```python
from build123d import *

# Parameters (mm, degrees)
BOSS_EXTRUDE1_DEPTH = 6
BOSS_EXTRUDE4_DEPTH = 20
CUT_EXTRUDE2_DEPTH  = 15
CUT_EXTRUDE3_DEPTH  = 6
CHAMFER2_SIZE       = 2
CHAMFER2_SIZE2      = 3.464101615


with BuildPart() as part:
    # Sketch1 → Boss-Extrude1 (new body)
    with BuildSketch(Plane(origin=(0, 0, 0), x_dir=(1, 0, 0), z_dir=(0, 1, 0))):
        Polygon((16.25, 9.381941874), (0, 18.763883749), (-16.25, 9.381941874), (-16.25, -9.381941874), (0, -18.763883749), (16.25, -9.381941874), align=None)
        Polygon((11.25, 6.495190528), (0, 12.990381057), (-11.25, 6.495190528), (-11.25, -6.495190528), (0, -12.990381057), (11.25, -6.495190528), align=None, mode=Mode.SUBTRACT)
    extrude(amount=BOSS_EXTRUDE1_DEPTH)

    # Sketch5 → Boss-Extrude4 (add)
    with BuildSketch(Plane.XZ):
        Polygon((16.25, 9.381941874), (0, 18.763883749), (-16.25, 9.381941874), (-16.25, -9.381941874), (0, -18.763883749), (16.25, -9.381941874), align=None)
    extrude(amount=BOSS_EXTRUDE4_DEPTH)

    # Sketch6 → Cut-Extrude2 (cut)
    with BuildSketch(Plane.XZ.offset(20)):
        with BuildLine():
            Line((-2.618090908, 1.66), (-2.618090908, -1.66))
            ThreePointArc((-2.618090908, -1.66), (3.1, 0), (-2.618090908, 1.66))
        make_face()
    extrude(amount=-CUT_EXTRUDE2_DEPTH, mode=Mode.SUBTRACT)

    # Sketch7 → Cut-Extrude3 (cut)
    with BuildSketch(Plane(origin=(0, 6, 0), x_dir=(1, 0, 0), z_dir=(0, 1, 0))):
        Polygon((-6.495190528, 11.25), (-12.990381057, 0), (-6.495190528, -11.25), (6.495190528, -11.25), (12.990381057, 0), (6.495190528, 11.25), align=None)
    extrude(amount=-CUT_EXTRUDE3_DEPTH, mode=Mode.SUBTRACT)

    # Chamfer2
    chamfer2_edges = [part.edges().sort_by_distance(p)[0] for p in [
        (4.754809472, 6, 11.25),
        (7.365381057, 6, 9.742785793),
        (11.25, 6, 4.754809472),
        (9.742785793, 6, -7.365381057),
        (-1.507214207, 6, -12.120190528),
        (-11.25, 6, -4.754809472),
        (-9.742785793, 6, 7.365381057),
        (1.507214207, 6, 12.120190528),
        (9.742785793, 6, 7.365381057),
        (-1.507214207, 6, 12.120190528),
        (-11.25, 6, 4.754809472),
        (-9.742785793, 6, -7.365381057),
        (1.507214207, 6, -12.120190528),
        (11.25, 6, -4.754809472),
        (12.120190528, 6, 1.507214207),
        (12.120190528, 6, -1.507214207),
        (7.365381057, 6, -9.742785793),
        (4.754809472, 6, -11.25),
        (-4.754809472, 6, -11.25),
        (-7.365381057, 6, -9.742785793),
        (-12.120190528, 6, -1.507214207),
        (-12.120190528, 6, 1.507214207),
        (-7.365381057, 6, 9.742785793),
        (-4.754809472, 6, 11.25),
    ]]
    chamfer2_side = [part.faces().sort_by_distance(p)[0] for p in [
        (7.87677715, 6, -13.642978223),
    ]]
    chamfer(chamfer2_edges, length=CHAMFER2_SIZE, length2=CHAMFER2_SIZE2, reference=chamfer2_side[0])


solid = part.part
```
Model file for the job. Use its own axes, mm. A direction names the side the tool comes from. Coordinates: 2 decimals unless noted, no trailing zeros. Write each loop counter-clockwise with the first axis right and the second up, starting at its lowest first coordinate (ties: lowest second). Pieces come first, ordered by that corner, then holes. Notation, with made-up numbers: (74, -16.5) - (120, -16.5) arc R24 cw to (120, 2.5) - close; hole circle Ø8 at (32, 37). An arc over 180 degrees is marked (long way). Use a Markdown table: item, result. Add a question column.
Item 1: Band-saw the part on B-B, the plane y = -0.5. Write the cut outline in (x, z).
Item 2: Band-saw the part on C-C, the plane x = -14. Write the cut outline in (y, z).
Item 3: Band-saw the part on D-D, the plane z = 1. Write the cut outline in (x, y).
Item 4: Two-plate mould, pull along Z, no slides. Class faces 3 (the face through (5.365, 4.244, -12.236)), 4 (the face through (-16.25, -7, 0)): pulls with the +Z half, pulls with the -Z half, needs draft (parallel to the pull), parting line crosses it, or undercut.
Item 5: Band-saw the part on A-A, the plane y = -17.5. Write the cut outline in (x, z).
Item 6: Drop flat-ended pins along their axis: pin 1 (2 mm diameter, centred on x = -4.5, y = -0.5, fed in from +Z); pin 2 (2 mm diameter, centred on x = 1.5, y = -8.5, fed in from -Z); pin 3 (8 mm diameter, centred on x = 6, y = -2, fed in from +Z). Give the stop position or say it passes through.
Item 7: Drill centre lines: line 1 along Z through (x, y) = (0, -9.25); line 2 along X through (y, z) = (-13, 0); line 3 along Y through (x, z) = (2, -2). Where is each one in solid material? Low to high.
Item 8: 3-axis set-ups, long thin cutter, end or side, ignore diameter. For faces 1 (the face through (-2.618, -13, 0)), 2 (the face through (7.914, 4.244, 10.764)): which of +Z, -Z, +X, -X, +Y, -Y reach the whole face in a straight line?
A:
| question | item | result |
|---|---|---|
| 1 | outline | (-16.25, -9.38) - (0, -18.76) - (16.25, -9.38) - (16.25, 9.38) - (0, 18.76) - (-16.25, 9.38) - close |
| 2 | outline | (-20, -10.68) - (6, -10.68) - (6, -2.25) - (4.05, 0) - (6, 2.25) - (6, 10.68) - (-20, 10.68) - close |
| 3 | outline | (-16.25, -20) - (-2.62, -20) - (-2.62, -5) - (2.93, -5) - (2.93, -20) - (16.25, -20) - (16.25, 6) - (14.72, 6) - (12.41, 2.54) - (12.41, 0) - (-12.41, 0) - (-12.41, 2.54) - (-14.72, 6) - (-16.25, 6) - close |
| 4 | face 3 | undercut |
| 4 | face 4 | needs draft |
| 5 | outline | (-16.25, -9.38) - (0, -18.76) - (16.25, -9.38) - (16.25, 9.38) - (0, 18.76) - (-16.25, 9.38) - close; hole (-2.62, -1.66) arc R3.1 ccw (long way) to (-2.62, 1.66) - close |
| 6 | pin 1 | stops at z = 16.74 |
| 6 | pin 2 | stops at z = -18.48 |
| 6 | pin 3 | stops at z = 17.61 |
| 7 | line 1 | z = -18.76 to -3.1, 3.1 to 18.76 |
| 7 | line 2 | x = -16.25 to -2.62, 3.1 to 16.25 |
| 7 | line 3 | y = -5 to 0 |
| 8 | face 1 | -Y |
| 8 | face 2 | +Y |
